Part model, mm, in its own coordinate system. A direction names the side the tool comes from. Round coordinates to 2 decimals unless told otherwise and drop trailing zeros.
```python
from build123d import *

# Parameters (mm, degrees)
SKETCH_1_W             = 23.5
SKETCH_1_H             = 12
EXTRUDE_1_DEPTH        = 650.5
HOLE_WIZARD_M6_1_D     = 5
HOLE_WIZARD_M6_1_DEPTH = 19
HOLE_WIZARD_M6_1_TIP   = 1.502151548
HOLE_WIZARD_M6_2_D     = 5
HOLE_WIZARD_M6_2_DEPTH = 19
HOLE_WIZARD_M6_2_TIP   = 1.502151548
HOLE_WIZARD_M4_1_D     = 3.3
HOLE_WIZARD_M4_1_DEPTH = 11.5
HOLE_WIZARD_M4_1_TIP   = 0.991420021


with BuildPart() as part:
    # 草图1 → 凸台-拉伸1 (new, symmetric)
    with BuildSketch(Plane(origin=(0, 0, 0), x_dir=(0, 0, -1), z_dir=(1, 0, 0))):
        Polygon((-15, 15), (-11.5, 15), (-11.5, 13.5), (-11, 13.5), (-11, 12), (-9.5, 12), (-9.5, 15), (-8, 15), (-8, 12.5), (-5, 12.5), (-5, 15), (5, 15), (5, 12.5), (8, 12.5), (8, 15), (9.5, 15), (9.5, 12), (11, 12), (11, 13.5), (11.5, 13.5), (11.5, 15), (15, 15), (15, 8), (12.5, 8), (12.5, 5), (15, 5), (15, -5), (12.5, -5), (12.5, -8), (15, -8), (15, -15), (11.5, -15), (11.5, -13.5), (11, -13.5), (11, -12), (9.5, -12), (9.5, -15), (8, -15), (8, -12.5), (5, -12.5), (5, -15), (-5, -15), (-5, -12.5), (-8, -12.5), (-8, -15), (-9.5, -15), (-9.5, -12), (-11, -12), (-11, -13.5), (-11.5, -13.5), (-11.5, -15), (-15, -15), align=None)
        with BuildLine():
            Line((12, -10.5), (12, -8.5))
            ThreePointArc((12, -8.5), (11.853553391, -8.146446609), (11.5, -8))
            Line((11.5, -8), (-11.5, -8))
            ThreePointArc((-11.5, -8), (-11.853553391, -8.146446609), (-12, -8.5))
            Line((-12, -8.5), (-12, -10.5))
            ThreePointArc((-12, -10.5), (-11.853553391, -10.853553391), (-11.5, -11))
            Line((-11.5, -11), (11.5, -11))
            ThreePointArc((11.5, -11), (11.853553391, -10.853553391), (12, -10.5))
        make_face(mode=Mode.SUBTRACT)
        with BuildLine():
            Line((-11.5, 11), (11.5, 11))
            ThreePointArc((11.5, 11), (11.853553391, 10.853553391), (12, 10.5))
            Line((12, 10.5), (12, 8.5))
            ThreePointArc((12, 8.5), (11.853553391, 8.146446609), (11.5, 8))
            Line((11.5, 8), (-11.5, 8))
            ThreePointArc((-11.5, 8), (-11.853553391, 8.146446609), (-12, 8.5))
            Line((-12, 8.5), (-12, 10.5))
            ThreePointArc((-12, 10.5), (-11.853553391, 10.853553391), (-11.5, 11))
        make_face(mode=Mode.SUBTRACT)
        Rectangle(SKETCH_1_W, SKETCH_1_H, mode=Mode.SUBTRACT)
    extrude(amount=EXTRUDE_1_DEPTH, both=True)

    # M6 螺纹孔1
    with Locations(Plane(origin=(0, 15, 0), x_dir=(1, 0, 0), z_dir=(0, 1, 0))):
        with Locations((-630.5, 0), (-615.5, 0), (615.5, 0), (630.5, 0), (-211.5, 0), (-157.5, 0), (83.5, 0), (137.5, 0)):
            Hole(HOLE_WIZARD_M6_1_D / 2, depth=HOLE_WIZARD_M6_1_DEPTH)
            with Locations((0, 0, -(HOLE_WIZARD_M6_1_DEPTH + HOLE_WIZARD_M6_1_TIP / 2))):  # 118° drill point
                Cone(0, HOLE_WIZARD_M6_1_D / 2, HOLE_WIZARD_M6_1_TIP, mode=Mode.SUBTRACT)

    # M6 螺纹孔2
    with Locations(Plane(origin=(0, 0, -15), x_dir=(-1, 0, 0), z_dir=(0, 0, -1))):
        with Locations((133.5, 0), (-6.5, 0)):
            Hole(HOLE_WIZARD_M6_2_D / 2, depth=HOLE_WIZARD_M6_2_DEPTH)
            with Locations((0, 0, -(HOLE_WIZARD_M6_2_DEPTH + HOLE_WIZARD_M6_2_TIP / 2))):  # 118° drill point
                Cone(0, HOLE_WIZARD_M6_2_D / 2, HOLE_WIZARD_M6_2_TIP, mode=Mode.SUBTRACT)

    # M4 螺纹孔1
    with Locations(Plane(origin=(0, 0, -15), x_dir=(-1, 0, 0), z_dir=(0, 0, -1))):
        with Locations((-312, 0)):
            Hole(HOLE_WIZARD_M4_1_D / 2, depth=HOLE_WIZARD_M4_1_DEPTH)
            with Locations((0, 0, -(HOLE_WIZARD_M4_1_DEPTH + HOLE_WIZARD_M4_1_TIP / 2))):  # 118° drill point
                Cone(0, HOLE_WIZARD_M4_1_D / 2, HOLE_WIZARD_M4_1_TIP, mode=Mode.SUBTRACT)


solid = part.part
```
Q1. Which spindle directions (+Z, -Z, +X, -X, +Y, -Y) get a long thin tool onto all of the face, cutting with end or side? Do faces 4 (the flat face through (9, 11, 0)), 5 (the flat face through (-650.5, 7, 0)). Say none if no direction does.
Values follow:
face 4: +X, -X
face 5: +Z, -Z, -X, +Y, -Y
Q2. Mould opens along Z. For faces 1 (the flat face through (9, 6, 0)), 2 (the flat face through (650.5, 7, 0)), 3 (the flat face through (9, 0, 15)) say: +Z half, -Z half, draft (parallel to the pull), parting line (faces both ways), or undercut.
Values follow:
face 1: undercut
face 2: draft
face 3: +Z half
Q3. Drop flat-ended pins along their axis: pin 1 (3 mm diameter, centred on x = 630.5, z = 0, fed in from +Y); pin 2 (1.5 mm diameter, centred on x = -18.5, y = -6, fed in from -Z); pin 3 (2 mm diameter, centred on x = 312, y = 0, fed in from -Z). Give the stop position or say it passes through.
Values follow:
pin 1: stops at y = -6
pin 2: stops at z = -12.5
pin 3: stops at z = 11.75
Q4. Cut at A-A on x = -489. State how many separate pieces and enclosed holes the cut face has, plus the area to 3 significant figures.
Values follow:
separate pieces: 1
enclosed holes: 3
area: 408 mm2
Q5. Wall check: L1, parallel to Z at x = -157.5, y = 13.4; L2, parallel to Y at x = 223, z = 3.5; L3, parallel to Z at x = 137.5, y = 12.15. Give the ranges that are in metal, low to high.
Values follow:
L1: z = -15 to -11, -9.5 to -8, -5 to -2.5, 2.5 to 5, 8 to 9.5, 11 to 15
L2: y = -15 to -11, -8 to -6, 6 to 8, 11 to 15
L3: z = -15 to -11, -9.5 to -2.5, 2.5 to 9.5, 11 to 15
